Build history of the part. All positions in model axes, mm. A direction names the side the tool comes from. Round coordinates to 2 decimals unless told otherwise and drop trailing zeros. Write each loop counter-clockwise with the first axis right and the second up, starting at its lowest first coordinate (ties: lowest second). Pieces come first, ordered by that corner, then holes.
1) Pull direction X, two halves, no side cores. Call faces 1 (the cylindrical face through (-37.69, -0.96, 32.18)), 2 (the cylindrical face through (47, 0, 11)), 3 (the flat face through (-60, 0, 10)): +X half, -X half, draft (parallel to the pull), parting line (faces both ways), or undercut.
2) Saw through at C-C (z = 17). Write the cut outline in (x, y).
3) Saw through at A-A (x = -15). Write the cut outline in (y, z).
4) Saw through at D-D (x = 57.5). Write the cut outline in (y, z), plus the area to 3 significant figures.
5) Flat gauge pins, fed straight in: pin 1 (0.9 mm diameter, centred on x = -57, y = -1, fed in from +Z); pin 2 (1.5 mm diameter, centred on y = 1, z = -15, fed in from +X); pin 3 (2.5 mm diameter, centred on y = 1, z = 19.5, fed in from +X). Where does each tip first touch, or does it go through?
6) Wall check: probe 1 along Z at (x, y) = (-40, -0.5); probe 2 along Z at (x, y) = (29, -1.85); probe 3 along X at (y, z) = (0.1, -34). Give the ranges that are in metal, low to high.
7) Saw through at B-B (z = 0). Write the cut outline in (x, y), plus the area to 3 significant figures.
8) Which spindle directions (+Z, -Z, +X, -X, +Y, -Y) get a long thin tool onto all of the face, cutting with end or side? Do faces 4 (the flat face through (39, 0, 37)), 5 (the flat face through (45, 0, -20)), 6 (the flat face through (-56, -1, -2)). Say none if no direction does.
from build123d import *

# Parameters (mm, degrees)
F1_DEPTH  = 2.5
F2_T      = -2
F5_SIZE   = 1
F6_W      = 75
F6_H      = 5
F7_DEPTH  = 39.501
F8_W      = 2
F8_H      = 5.8988734534
F9_DEPTH  = 6
F12_R     = 5
F13_DEPTH = 5
F15_D     = 6


with BuildPart() as f1:
    # F0 (on Front) → F1 (new body, symmetric)
    with BuildSketch(Plane.XZ):
        with BuildLine():
            Line((0, 10), (0, 0))
            Line((0, 0), (70, 0))
            Line((70, 0), (70, 10))
            Line((70, 10), (50, 10))
            ThreePointArc((50, 10), (46.4644660941, 11.4644660941), (45, 15))
            Line((45, 15), (45, 25))
            Line((45, 25), (35, 25))
            Line((35, 25), (35, 15))
            ThreePointArc((35, 15), (33.5355339059, 11.4644660941), (30, 10))
            Line((30, 10), (8.4090904464, 10))
            Line((8.4090904464, 10), (0, 10))
        make_face()
    extrude(amount=F1_DEPTH, both=True)

    # F2
    f2_openings = [f1.faces().sort_by_distance(p)[0] for p in [
        (35.933685, -2.5, 7.254637),
    ]]
    offset(amount=F2_T, openings=f2_openings)

    # F3 (on Front) → F4 (revolve)
    with BuildSketch(Plane.XZ):
        Polygon((37, 25), (40, 25), (40, 39.5), (37, 39.5), (37, 37.5), (37.5, 37.5), (37.5, 27), (37, 27), align=None)
    revolve(axis=Axis((40, 0, 32.25), (0, 0, -1)))

    # F5
    f5_edges = [f1.edges().sort_by_distance(p)[0] for p in [
        (43, 0, 39.5),
    ]]
    chamfer(f5_edges, length=F5_SIZE)

    # F6 (on face) → F7 (intersect, through all)
    with BuildSketch(Plane.XY.offset(39.5)):
        with Locations((35.0839576957, 0)):
            Rectangle(F6_W, F6_H)
    extrude(amount=-F7_DEPTH, mode=Mode.INTERSECT)

    # F8 (on face) → F9 (cut)
    with BuildSketch(Plane.XY.offset(39.5)):
        with Locations((40, 0)):
            Rectangle(F8_W, F8_H)
    extrude(amount=-F9_DEPTH, mode=Mode.SUBTRACT)

    # F10: F1 across plane


with BuildPart() as f1_1:
    add(f1.part)
    add(f1.part.mirror(Plane.XY))

    # F11: F1 across plane


with BuildPart() as f1_2:
    add(f1_1.part)
    add(f1_1.part.mirror(Plane.YZ))

    # F12 (on face) → F13 (join, through all)
    with BuildSketch(Plane.XZ.offset(2.5)):
        with Locations((-40, 0)):
            Circle(F12_R)
        with Locations((-15, 0)):
            Circle(F12_R)
    extrude(amount=-F13_DEPTH)

    # F15 (through all)
    with Locations(Plane.XZ.offset(2.5)):
        with Locations((-40, 0), (-15, 0)):
            Hole(F15_D / 2)


solid = f1_2.part
Evaluation:
1. face 1: undercut
1. face 2: +X half
1. face 3: draft
2. outline: (-45, -2.5) - (-43, -2.5) - (-43, 0.5) - (-37, 0.5) - (-37, -2.5) - (-35, -2.5) - (-35, 2.5) - (-45, 2.5) - close; (35, -2.5) - (37, -2.5) - (37, 0.5) - (43, 0.5) - (43, -2.5) - (45, -2.5) - (45, 2.5) - (35, 2.5) - close
3. outline: (-2.5, -10) - (2.5, -10) - (2.5, -3) - (-2.5, -3) - (-2.5, -5) - (0.5, -5) - (0.5, -8) - (-2.5, -8) - close; (-2.5, 3) - (2.5, 3) - (2.5, 10) - (-2.5, 10) - (-2.5, 8) - (0.5, 8) - (0.5, 5) - (-2.5, 5) - close
4. outline: (-2.5, -10) - (2.5, -10) - (2.5, 10) - (-2.5, 10) - (-2.5, 8) - (0.5, 8) - (0.5, 2) - (-2.5, 2) - (-2.5, -2) - (0.5, -2) - (0.5, -8) - (-2.5, -8) - close
4. area: 64.0 mm2
5. pin 1: stops at z = 10
5. pin 2: stops at x = 45.06
5. pin 3: stops at x = 45
6. probe 1: z = -33.5 to -23, -5 to -3, 3 to 5, 23 to 33.5
6. probe 2: z = -10 to -8, -2 to 2, 8 to 10
6. probe 3: x = -42.5 to -41, -39 to -37.5, 37.5 to 39, 41 to 42.5
7. outline: (-70, -2.5) - (-43, -2.5) - (-43, 2.5) - (-70, 2.5) - close; (-37, -2.5) - (-18, -2.5) - (-18, 2.5) - (-37, 2.5) - close; (-12, -2.5) - (70, -2.5) - (70, 2.5) - (-12, 2.5) - close
7. area: 640 mm2
8. face 4: +Z, +Y, -Y
8. face 5: -Z, +X, +Y, -Y
8. face 6: -Y
